The listing builds one solid part. Answer for the finished solid, in the listing's coordinates (mm). A direction names the side the tool comes from. Coordinates: 2 decimals unless noted, no trailing zeros. Loops run counter-clockwise (first coordinate to the right, second up) from the corner with the lowest first, then second, coordinate; pieces in that order, holes last. Notation, with made-up numbers: (77, 89.5) - (104, 89.5) arc R6 cw to (104, 99.5) - close; hole circle Ø8 at (-34, 27.25). An arc over 180 degrees is marked (long way). Put each result on its own line as item: value.
```python
from build123d import *

# Parameters (mm, degrees)
ESQUISSE1_W              = 50
ESQUISSE1_H              = 30
BOSS_EXTRU_1_DEPTH       = 40
ESQUISSE2_W              = 7
ESQUISSE2_H              = 7
ENL_V_MAT_EXTRU_1_DEPTH  = 41
ESQUISSE3_W              = 8
ESQUISSE3_H              = 10
ENL_V_MAT_EXTRU_2_DEPTH  = 41
ESQUISSE5_W              = 34.9
ESQUISSE5_H              = 30
ENL_V_MAT_EXTRU_4_DEPTH  = 35
ESQUISSE7_R              = 5.5
ESQUISSE7_R_2            = 1.8
ENL_V_MAT_EXTRU_6_DEPTH  = 41
BOSS_EXTRU_2_DEPTH       = 5
ESQUISSE10_R             = 2.1
ENL_V_MAT_EXTRU_7_DEPTH  = 31
ESQUISSE11_R             = 4
ENL_V_MAT_EXTRU_8_DEPTH  = 1
ENL_V_MAT_EXTRU_9_DEPTH  = 6
CONG_2_R                 = 2
ESQUISSE14_W             = 13
ESQUISSE14_H             = 12
ENL_V_MAT_EXTRU_10_DEPTH = 41
ESQUISSE15_W             = 40
ESQUISSE15_H             = 5
BOSS_EXTRU_3_DEPTH       = 30
ESQUISSE16_R             = 2.2
ENL_V_MAT_EXTRU_11_DEPTH = 6
ESQUISSE17_R             = 4
ENL_V_MAT_EXTRU_12_DEPTH = 1
CHANFREIN1_SIZE          = 20
CHANFREIN1_SIZE2         = 16
CONG_3_R                 = 10
CHANFREIN2_SIZE          = 35
CHANFREIN2_SIZE2         = 12
CONG_4_R                 = 10


with BuildPart() as part:
    # Esquisse1 → Boss.-Extru.1 (new body)
    with BuildSketch(Plane.XY):
        Rectangle(ESQUISSE1_W, ESQUISSE1_H)
    extrude(amount=BOSS_EXTRU_1_DEPTH)

    # Esquisse2 → Enlèv. mat.-Extru.1 (cut, through all)
    with BuildSketch(Plane.XY.offset(40)):
        with Locations((15.5, -6.5)):
            Rectangle(ESQUISSE2_W, ESQUISSE2_H)
        with Locations((15.5, 6.5)):
            Rectangle(ESQUISSE2_W, ESQUISSE2_H)
    extrude(amount=-ENL_V_MAT_EXTRU_1_DEPTH, mode=Mode.SUBTRACT)

    # Esquisse3 → Enlèv. mat.-Extru.2 (cut, through all)
    with BuildSketch(Plane.XY.offset(40)):
        with Locations((21, 0)):
            Rectangle(ESQUISSE3_W, ESQUISSE3_H)
    extrude(amount=-ENL_V_MAT_EXTRU_2_DEPTH, mode=Mode.SUBTRACT)

    # Esquisse5 → Enlèv. mat.-Extru.4 (cut)
    with BuildSketch(Plane.XY.offset(40)):
        with Locations((-7.55, 0)):
            Rectangle(ESQUISSE5_W, ESQUISSE5_H)
    extrude(amount=-ENL_V_MAT_EXTRU_4_DEPTH, mode=Mode.SUBTRACT)

    # Esquisse7 → Enlèv. mat.-Extru.6 (cut, through all)
    with BuildSketch(Plane(origin=(0, 0, 0), x_dir=(-1, 0, 0), z_dir=(0, 0, -1))):
        with Locations((9, 0)):
            Circle(ESQUISSE7_R)
        with Locations((22, 0)):
            Circle(ESQUISSE7_R_2)
        with Locations((-4, 0)):
            Circle(ESQUISSE7_R_2)
    extrude(amount=-ENL_V_MAT_EXTRU_6_DEPTH, mode=Mode.SUBTRACT)

    # Esquisse9 → Boss.-Extru.2 (add)
    with BuildSketch(Plane.XZ.offset(15)):
        Polygon((9.9, 40), (-6.1, 40), (-15.1, 5), (9.9, 5), align=None)
    extrude(amount=-BOSS_EXTRU_2_DEPTH)

    # Esquisse10 → Enlèv. mat.-Extru.7 (cut, through all)
    with BuildSketch(Plane.XZ.offset(15)):
        with Locations((5, 20)):
            Circle(ESQUISSE10_R)
    extrude(amount=-ENL_V_MAT_EXTRU_7_DEPTH, mode=Mode.SUBTRACT)

    # Esquisse11 → Enlèv. mat.-Extru.8 (cut)
    with BuildSketch(Plane(origin=(0, -10, 0), x_dir=(1, 0, 0), z_dir=(0, 1, 0))):
        with Locations((5, -20)):
            Circle(ESQUISSE11_R)
    extrude(amount=-ENL_V_MAT_EXTRU_8_DEPTH, mode=Mode.SUBTRACT)

    # Esquisse13 → Enlèv. mat.-Extru.9 (cut, through all)
    with BuildSketch(Plane.XY.offset(5)):
        Polygon((-15.1, -15), (-15.1, -10), (-25, -5), (-25, -15), align=None)
        Polygon((-25, 5), (-15.1, 10), (9.9, 15), (-25, 15), align=None)
    extrude(amount=-ENL_V_MAT_EXTRU_9_DEPTH, mode=Mode.SUBTRACT)

    # Congé2
    cong_2_edges = [part.edges().sort_by_distance(p)[0] for p in [
        (-6.1, -12.5, 40),
        (-25, -5, 2.5),
        (-25, 5, 2.5),
        (-15.1, 10, 2.5),
    ]]
    fillet(cong_2_edges, radius=CONG_2_R)

    # Esquisse14 → Enlèv. mat.-Extru.10 (cut, through all)
    with BuildSketch(Plane.XY.offset(40)):
        with Locations((18.5, 9)):
            Rectangle(ESQUISSE14_W, ESQUISSE14_H)
    extrude(amount=-ENL_V_MAT_EXTRU_10_DEPTH, mode=Mode.SUBTRACT)

    # Esquisse15 → Boss.-Extru.3 (add)
    with BuildSketch(Plane(origin=(25, 0, 0), x_dir=(0, 0, -1), z_dir=(1, 0, 0))):
        with Locations((-20, -12.5)):
            Rectangle(ESQUISSE15_W, ESQUISSE15_H)
    extrude(amount=BOSS_EXTRU_3_DEPTH)

    # Esquisse16 → Enlèv. mat.-Extru.11 (cut, through all)
    with BuildSketch(Plane(origin=(0, -10, 0), x_dir=(1, 0, 0), z_dir=(0, 1, 0))):
        with Locations((45, -20)):
            Circle(ESQUISSE16_R)
    extrude(amount=-ENL_V_MAT_EXTRU_11_DEPTH, mode=Mode.SUBTRACT)

    # Esquisse17 → Enlèv. mat.-Extru.12 (cut)
    with BuildSketch(Plane(origin=(0, -10, 0), x_dir=(1, 0, 0), z_dir=(0, 1, 0))):
        with Locations((45, -20)):
            Circle(ESQUISSE17_R)
    extrude(amount=-ENL_V_MAT_EXTRU_12_DEPTH, mode=Mode.SUBTRACT)

    # Chanfrein1
    chanfrein1_edges = [part.edges().sort_by_distance(p)[0] for p in [
        (55, -12.5, 40),
    ]]
    chanfrein1_side = [part.faces().sort_by_distance(p)[0] for p in [
        (22.378363324, -9.30070091, 40),
    ]]
    chamfer(chanfrein1_edges, length=CHANFREIN1_SIZE, length2=CHANFREIN1_SIZE2, reference=chanfrein1_side[0])

    # Congé3
    cong_3_edges = [part.edges().sort_by_distance(p)[0] for p in [
        (55, -12.5, 24),
    ]]
    fillet(cong_3_edges, radius=CONG_3_R)

    # Chanfrein2
    chanfrein2_edges = [part.edges().sort_by_distance(p)[0] for p in [
        (10.95, 15, 40),
    ]]
    chanfrein2_side = [part.faces().sort_by_distance(p)[0] for p in [
        (10.95, 15, 20),
    ]]
    chamfer(chanfrein2_edges, length=CHANFREIN2_SIZE, length2=CHANFREIN2_SIZE2, reference=chanfrein2_side[0])

    # Congé4
    cong_4_edges = [part.edges().sort_by_distance(p)[0] for p in [
        (35, -12.5, 40),
    ]]
    fillet(cong_4_edges, radius=CONG_4_R)


solid = part.part
```
1) The part is cut by section C-C (y = 0). Give the vertices of the cut face in (x, z), and give its area (4 significant figures).
Found:
outline: (-25, 0) - (-23.8, 0) - (-23.8, 5) - (-25, 5) - close; (-20.2, 0) - (-14.5, 0) - (-14.5, 5) - (-20.2, 5) - close; (-3.5, 0) - (2.2, 0) - (2.2, 5) - (-3.5, 5) - close; (5.8, 0) - (17, 0) - (17, 40) - (9.9, 40) - (9.9, 5) - (5.8, 5) - close
area: 367.5 mm^2
2) The part is cut by section D-D (z = 20). State how many separate pieces and enclosed holes the cut face has, and give its area (3 significant figures).
Found:
separate pieces: 3
enclosed holes: 0
area: 382 mm^2
3) For a pull along X with two mould halves and no side action, classify faces 4 (the face through (12, 8, 16)), 5 (the face through (6.13, -13.03, 21.77)), 6 (the face through (-19.44, -7.81, 2.54)), 7 (the face through (7, -11, 22)) as pulls with the +X half, pulls with the -X half, needs draft (parallel to the pull), parting line crosses it, or undercut.
Found:
face 4: pulls with the +X half
face 5: undercut
face 6: pulls with the -X half
face 7: undercut
4) Straight lines are drawn through the part: L1, parallel to Z at x = 5, y = -11.75; L2, parallel to X at y = -10.45, z = 20; L3, parallel to X at y = -7.5, z = 13.5. For each, find the intervals that lie inside material, in ascending order. Write a range as [from, to].
Found:
L1: z = [0, 17.9], [22.1, 40]
L2: x = [-11.24, 1], [9, 41], [49, 54.97]
L3: x = [9.9, 12], [19, 25]
5) The part is cut by section A-A (y = -7). Give the vertices of the cut face in (x, z), and give its area (3 significant figures).
Found:
outline: (-21.04, 0) - (12, 0) - (12, 40) - (9.9, 40) - (9.9, 5) - (-21.04, 5) - close; (19, 0) - (25, 0) - (25, 40) - (19, 40) - close
area: 479 mm^2
6) For faces 1 (the face through (47, -11, 22)), 2 (the face through (-15.1, -13, 3)), 3 (the face through (40, -10, 16)), determine the directions among +Z, -Z, +X, -X, +Y, -Y from which every point of the face is accessible in a straight line to the end or side of a thin tool.
Found:
face 1: +Y
face 2: +Z, -Z, -X, -Y
face 3: +Z, -Z, +X, +Y
7) The part is cut by section B-B (x = 45). Give the vertices of the cut face in (y, z), and give its area (3 significant figures).
Found:
outline: (-15, 0) - (-10, 0) - (-10, 16) - (-11, 16) - (-11, 17.8) - (-15, 17.8) - close; (-15, 22.2) - (-11, 22.2) - (-11, 24) - (-10, 24) - (-10, 32) - (-15, 32) - close
area: 134 mm^2
8) Each of these flat-tipped pins is pushed along its axis until it touches: pin 1 (6 mm diameter, centred on x = 26.5, z = 35, fed in from +Y); pin 2 (3.5 mm diameter, centred on y = -7, z = 26.5, fed in from +X); pin 3 (4 mm diameter, centred on y = -11.5, z = 2.5, fed in from -X). Where does it stop, or does it pass through?
Found:
pin 1: stops at y = -5
pin 2: stops at x = 25
pin 3: stops at x = -16.09
